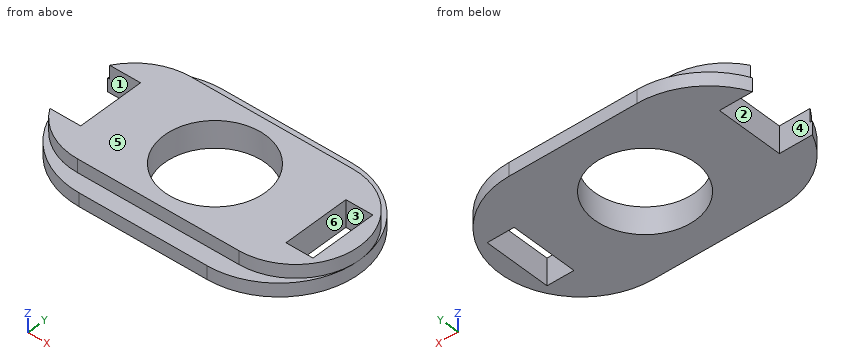
```python
from build123d import *

# Parameters (mm, degrees)
EXTRUSION1_DEPTH        = 2
EXTRUSION4_DEPTH        = 2
ESQUISSE3_R             = 7.5
ESQUISSE3_W             = 4
ESQUISSE3_H             = 10
ESQUISSE3_W_2           = 6
ENL_V_MAT_EXTRU_1_DEPTH = 5


with BuildPart() as part:
    # Esquisse1 → Extrusion1 (new body)
    with BuildSketch(Plane.XY):
        with BuildLine():
            Line((-57.049073, 33.907042), (-38.049073, 33.907042))
            ThreePointArc((-38.049073, 33.907042), (-26.049073, 21.907042), (-38.049073, 9.907042))
            Line((-38.049073, 9.907042), (-57.049073, 9.907042))
            ThreePointArc((-57.049073, 9.907042), (-69.049073, 21.907042), (-57.049073, 33.907042))
        make_face()
    extrude(amount=EXTRUSION1_DEPTH)

    # Esquisse2 → Extrusion4 (add)
    with BuildSketch(Plane.XY.offset(2)):
        with BuildLine():
            Line((-59.549073, 31.407042), (-35.549073, 31.407042))
            ThreePointArc((-35.549073, 31.407042), (-26.049073, 21.907042), (-35.549073, 12.407042))
            Line((-35.549073, 12.407042), (-59.549073, 12.407042))
            ThreePointArc((-59.549073, 12.407042), (-69.049073, 21.907042), (-59.549073, 31.407042))
        make_face()
    extrude(amount=EXTRUSION4_DEPTH)

    # Esquisse3 → Enlèv. mat.-Extru.1 (cut, through all)
    with BuildSketch(Plane.XY.offset(4)):
        with Locations((-47.549073, 21.907042)):
            Circle(ESQUISSE3_R)
        with Locations((-30.549073, 21.907042)):
            Rectangle(ESQUISSE3_W, ESQUISSE3_H)
        with Locations((-66.049073, 21.907042)):
            Rectangle(ESQUISSE3_W_2, ESQUISSE3_H)
    extrude(amount=-ENL_V_MAT_EXTRU_1_DEPTH, mode=Mode.SUBTRACT)


solid = part.part
```
Design review of the part built by this model. Coordinates are the model's own, in mm. Face numbers are marked on the shaded views. A direction names the side the tool comes from. Round coordinates to 2 decimals unless told otherwise and drop trailing zeros. Write each loop counter-clockwise with the first axis right and the second up, starting at its lowest first coordinate (ties: lowest second). Pieces come first, ordered by that corner, then holes. Notation, with made-up numbers: (34, 86) -> (52, 86) arc R32 cw to (52, 112) -> close; hole circle Ø9 at (45, 2). An arc over 180 degrees is marked (long way). Answer in a Markdown table with one row per item.
Q1. To check wall thickness, follow L1, parallel to X at y = 22.75, z = 0.9; L2, parallel to X at y = 23.5, z = 3.75; L3, parallel to Z at x = -55.5, y = 32.25. State the ranges of each line that lie inside material, in increasing order. Write a range as [from, to].
The answers:
| item | result |
|---|---|
| L1 | [-63.05, -55], [-40.1, -32.55], [-28.55, -26.08] |
| L2 | [-63.05, -54.88], [-40.22, -32.55], [-28.55, -26.18] |
| L3 | [0, 2] |
Q2. Take a section at B-B, the plane x = -45. State the section outline as (y, z) points, then the cut area to 3 significant figures.
The answers:
| item | result |
|---|---|
| outline | (9.91, 0) -> (14.85, 0) -> (14.85, 4) -> (12.41, 4) -> (12.41, 2) -> (9.91, 2) -> close; (28.96, 0) -> (33.91, 0) -> (33.91, 2) -> (31.41, 2) -> (31.41, 4) -> (28.96, 4) -> close |
| area | 29.6 mm² |
Q3. Take a section at C-C, the plane y = 23.75. Count the separate pieces of the cut face and the enclosed holes in it, then the cut area to 3 significant figures.
The answers:
| item | result |
|---|---|
| separate pieces | 3 |
| enclosed holes | 0 |
| area | 73.2 mm² |
Q4. Take a section at D-D, the plane y = 16.5. State the section outline as (x, z) points.
The answers:
| item | result |
|---|---|
| outline | (-67.76, 0) -> (-52.75, 0) -> (-52.75, 4) -> (-67.36, 4) -> (-67.36, 2) -> (-67.76, 2) -> close; (-42.35, 0) -> (-27.34, 0) -> (-27.34, 2) -> (-27.74, 2) -> (-27.74, 4) -> (-42.35, 4) -> close |
Q5. Draft analysis for pull direction X (two halves, no side actions). For the marked faces 1, 2 and 3, state which applies: +X half, -X half, draft (parallel to the pull), parting line (faces both ways), or undercut.
The answers:
| item | result |
|---|---|
| face 1 | draft |
| face 2 | -X half |
| face 3 | undercut |
Q6. Take a section at A-A, the plane z = 1.5. State the section outline as (x, y) points.
The answers:
| item | result |
|---|---|
| outline | (-67.96, 16.91) arc R12 ccw to (-57.05, 9.91) -> (-38.05, 9.91) arc R12 ccw to (-38.05, 33.91) -> (-57.05, 33.91) arc R12 ccw to (-67.96, 26.91) -> (-63.05, 26.91) -> (-63.05, 16.91) -> close; hole circle Ø15 at (-47.55, 21.91); hole (-32.55, 16.91) -> (-28.55, 16.91) -> (-28.55, 26.91) -> (-32.55, 26.91) -> close |
Q7. Clearance check with flat-ended pins moving along their axes: pin 1 Ø2 at (x, y) = (-34.5, 19.5) entering from -Z; pin 2 Ø1.2 at (x, z) = (-31.5, 1.5) entering from -Y; pin 3 Ø2 at (x, z) = (-30.5, 2.5) entering from +Y; pin 4 Ø2 at (y, z) = (30.5, 0.5) entering from -X. State where each tip first meets the part, or that it passes through.
The answers:
| item | result |
|---|---|
| pin 1 | z = 0 |
| pin 2 | y = 11.49 |
| pin 3 | y = 31.87 |
| pin 4 | x = -66.34 |
Q8. For the marked faces 4, 5 and 6, list the 3-axis set-ups (+Z, -Z, +X, -X, +Y, -Y) from which the entire face can be reached by the end or side of a thin tool; tool diameter is ignored.
The answers:
| item | result |
|---|---|
| face 4 | +Z, -Z, -X |
| face 5 | +Z, +X, -X, +Y, -Y |
| face 6 | +Z, -Z |
